Could you check a few things on this drawing? It's one solid part, dimensions in mm from its lowest x, y, z. Give positions to 0.01 mm unless a question says otherwise; leave off trailing zeros. Loops run counter-clockwise (first coordinate to the right, second up) from the corner with the lowest first, then second, coordinate; pieces in that order, holes last. Notation, with made-up numbers: (-7, -27) -> (39, -27) arc R16 ccw to (39, 2) -> close; hole circle Ø1 at (83.5, 10.5). An arc over 180 degrees is marked (long way). One line per question, with ' | ' between items.
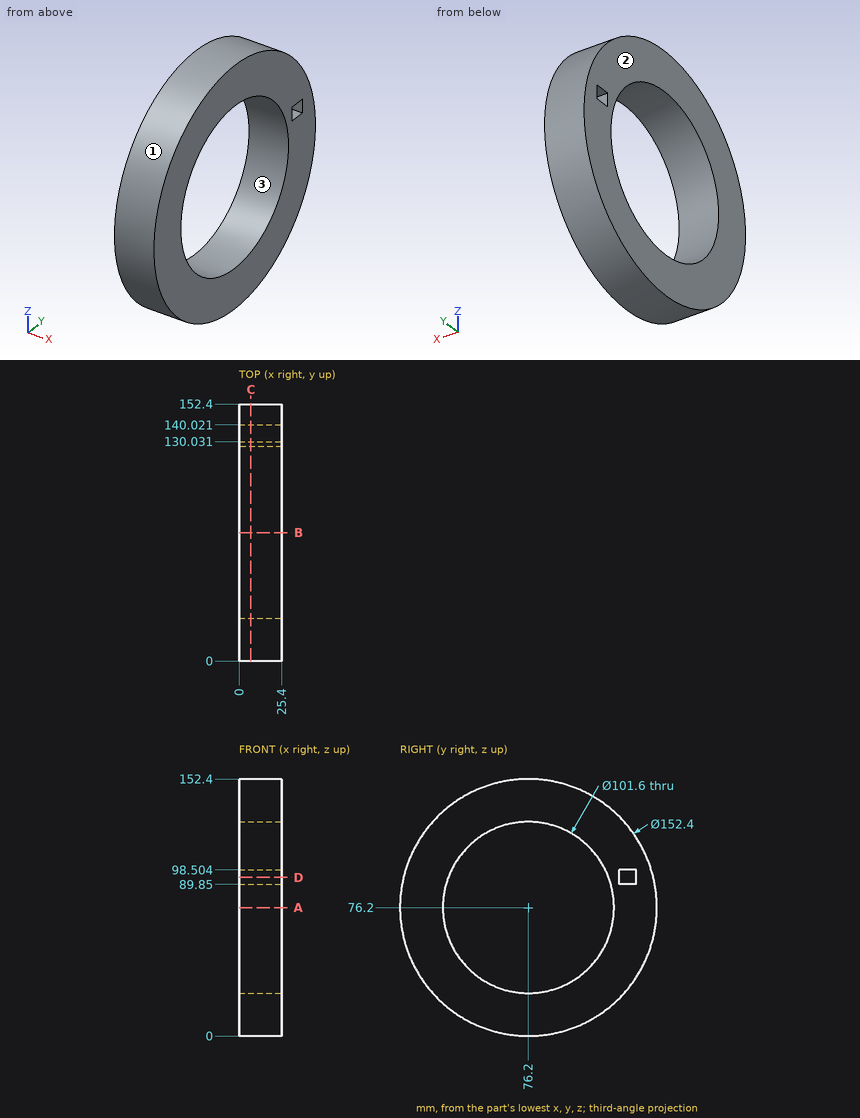
Q1. If I drill on probe 1 along Z at (x, y) = (9.25, 76.2); probe 2 along Z at (x, y) = (17, 123) (1 decimal); probe 3 along Y at (x, z) = (4.5, 38), over which ranges is the centre line in solid material (lowest first)? Write a range as from..to.
Entries:
probe 1: 0..25.4, 127..152.4 | probe 2: 16.1..56.4, 96..136.3 | probe 3: 10.27..42.71, 109.69..142.13
Q2. If we section it at C-C (x = 7): Write out the boundary of the cut face in (y, z).
Entries:
outline: circle Ø152.4 at (76.2, 76.2); hole circle Ø101.6 at (76.2, 76.2); hole (130.03, 89.85) -> (140.02, 89.85) -> (140.02, 98.5) -> (130.03, 98.5) -> close
Q3. If we section it at D-D (z = 94): Write out the boundary of the cut face in (x, y), plus the area to 3 significant figures.
Entries:
outline: (0, 2.11) -> (25.4, 2.11) -> (25.4, 28.62) -> (0, 28.62) -> close; (0, 123.78) -> (25.4, 123.78) -> (25.4, 130.03) -> (0, 130.03) -> close; (0, 140.02) -> (25.4, 140.02) -> (25.4, 150.29) -> (0, 150.29) -> close | area: 1,090 mm²
Q4. If we section it at A-A (z = 76.2): Write out the boundary of the cut face in (x, y).
Entries:
outline: (0, 0) -> (25.4, 0) -> (25.4, 25.4) -> (0, 25.4) -> close; (0, 127) -> (25.4, 127) -> (25.4, 152.4) -> (0, 152.4) -> close
Q5. If we mould it in two halves opening along Y, with no side actions, what happens to the marked faces 1, 2 and 3? For each: pulls with the +Y half, pulls with the -Y half, needs draft (parallel to the pull), parting line crosses it, or undercut.
Entries:
face 1: parting line crosses it | face 2: needs draft | face 3: undercut
Q6. For pin 1 Ø8 at (x, y) = (14, 79.5) entering from +Z; pin 2 Ø3 at (x, y) = (5.5, 44.5) entering from +Z; pin 3 Ø1 at (x, z) = (11.5, 67.5) entering from -Y, each with a flat end and sliding along its axis, tell me the tip position at first contact or that it passes through.
Entries:
pin 1: z = 152.4 | pin 2: z = 146.16 | pin 3: y = 0.44
